Can you work these out from the drawing? Everything is in mm from the part's minimum corner. Give positions to 0.01 mm unless a question says otherwise; leave off trailing zeros. Loops run counter-clockwise (first coordinate to the right, second up) from the corner with the lowest first, then second, coordinate; pieces in that order, holes last. Notation, with made-up numbers: (61.25, 60) - (83.25, 60) arc R28 cw to (83.25, 87) - close; hole circle Ø10 at (38, 28.5). An arc over 180 degrees is marked (long way). Answer in a Markdown table with one row per item.
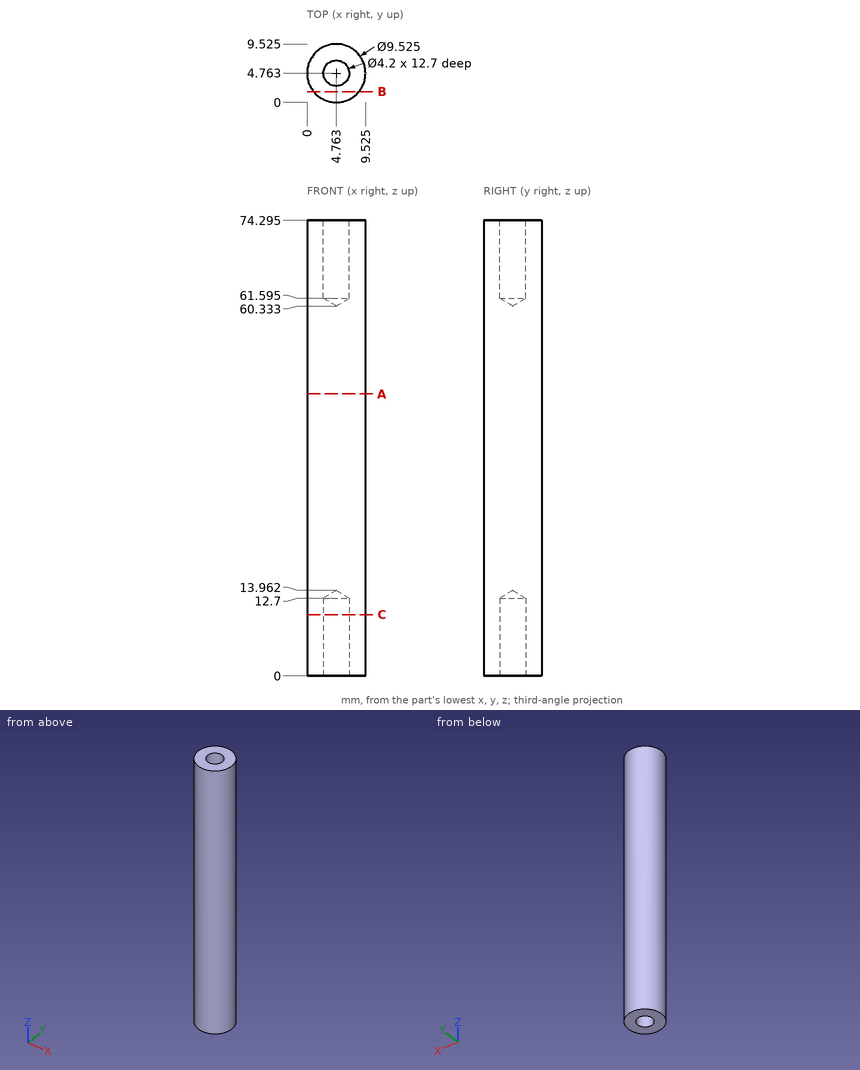
Q1. Imagine slicing it at B-B, the plane y = 1.75. Write out the boundary of the cut face in (x, z) (1 decimal), and give its area (3 significant figures).
Checked values:
| item | result |
|---|---|
| outline | (1.1, 0) - (8.5, 0) - (8.5, 74.3) - (1.1, 74.3) - close |
| area | 548 mm² |
Q2. Imagine slicing it at A-A, the plane z = 46. Write out the boundary of the cut face in (x, y) (1 decimal).
Checked values:
| item | result |
|---|---|
| outline | circle Ø9.5 at (4.8, 4.8) |
Q3. Imagine slicing it at C-C, the plane z = 10. Write out the boundary of the cut face in (x, y) (1 decimal).
Checked values:
| item | result |
|---|---|
| outline | circle Ø9.5 at (4.8, 4.8); hole circle Ø4.2 at (4.8, 4.8) |
Q4. If I drill on line 1 (Y direction, x = 4.5, z = 24.5); line 2 (X direction, y = 4, z = 5) (1 decimal); line 3 (Z direction, x = 5.5, y = 6) (1 decimal), over which ranges is the centre line in solid material (lowest first)? Write a range as [from, to].
Checked values:
| item | result |
|---|---|
| line 1 | y = [0.01, 9.52] |
| line 2 | x = [0.1, 2.8], [6.7, 9.5] |
| line 3 | z = [13.1, 61.2] |
Q5. For pin 1 (3 mm diameter, centred on y = 3.5, z = 54.5, fed in from -X); pin 2 (4 mm diameter, centred on x = 4.76, y = 4.76, fed in from +Z); pin 3 (1 mm diameter, centred on x = 7.5, z = 22.5, fed in from -Y); pin 4 (1.5 mm diameter, centred on x = 3.5, z = 20.5, fed in from +Y), each with a flat end and sliding along its axis, tell me the tip position at first contact or that it passes through.
Checked values:
| item | result |
|---|---|
| pin 1 | stops at x = 0 |
| pin 2 | stops at z = 61.54 |
| pin 3 | stops at y = 0.56 |
| pin 4 | stops at y = 9.5 |
